Autodesk Inventor part; units mm, degrees
ref_plane "YZ Plane" through (0, 0, 0) normal (1, 0, 0) x (0, 1, 0)
ref_plane "XZ Plane" through (0, 0, 0) normal (0, 1, 0) x (-1, 0, 0)
ref_plane "XY Plane" through (0, 0, 0) normal (0, 0, 1) x (1, 0, 0)
sketch "Sketch1" plane through (0, 0, 0) normal (0, 1, 0) x (-1, 0, 0)
  line L0 (-10, 22.5) -> (-10, -22.5)
  line L1 (-10, -22.5) -> (10, -22.5)
  line L2 (10, -22.5) -> (10, 22.5)
  line L3 (10, 22.5) -> (-10, 22.5)
  line L4 (-10, 22.5) -> (10, -22.5) construction
  line L5 (-10, -22.5) -> (10, 22.5) construction
  point P0 (0, 0)
  dimension "d0" = 45
  dimension "d1" = 20
extrude "Extrusion1" add sketch "Sketch1" along normal blind 2
sketch "Sketch2" plane through (0, 2, 0) normal (0, 1, 0) x (1, 0, 0)
  line L0 (7.5, -20) -> (7.5, 20)
  line L1 (7.5, 20) -> (-7.5, 20)
  line L2 (-7.5, 20) -> (-7.5, -20)
  line L3 (-7.5, -20) -> (7.5, -20)
  line L4 (7.5, -20) -> (-7.5, 20) construction
  line L5 (7.5, 20) -> (-7.5, -20) construction
  circle A0 centre (-7.5, -20) radius 1
  circle A1 centre (7.5, -20) radius 1
  circle A2 centre (7.5, 20) radius 1
  circle A3 centre (-7.5, 20) radius 1
  point P0 (0, 0)
  dimension "d25" = 40
  dimension "d26" = 15
  dimension "d27" = 2
  dimension "d28" = 2
  dimension "d29" = 2
  dimension "d30" = 2
extrude "Extrusion2" cut sketch "Sketch2" against normal blind 2 contours L3 A1 L0 | L0 A1 L3 | A2 L1 L0 | L0 L1 A2 | A0 L2 L3 | L3 L2 A0 | A3 L2 L1 | L1 L2 A3
sketch "Sketch3" plane through (0, 2, 0) normal (0, 1, 0) x (1, 0, 0)
  circle A0 centre (0, -13.5) radius 8
  circle A1 centre (0, 13.5) radius 8
  dimension "d33" = 16
  dimension "d34" = 16
extrude "Extrusion3" add sketch "Sketch3" along normal blind 13.8
fillet "Fillet1" radius 1 2 edges at (-8, 15.8, -13.5) (-8, 15.8, 13.5)
sketch "Sketch4" plane through (0, 15.8, 13.5) normal (0, 1, 0) x (1, 0, 0)
  circle A0 centre (0, 0) radius 8
  circle A1 centre (0, 27) radius 8
  circle A2 centre (0, 0) radius 6.5
  circle A3 centre (0, 27) radius 6.5
  dimension "d35" = 13
  dimension "d36" = 13
extrude "Extrusion4" cut sketch "Sketch4" against normal blind 1 contours A2 | A3
properties part number "HC-SR04 Sonar"
Can you work these out from the model? Positions are in its coordinate system, mm. A direction names the side the tool comes from. Give positions to 0.01 mm unless a question says otherwise; leave off trailing zeros. Loops run counter-clockwise (first coordinate to the right, second up) from the corner with the lowest first, then second, coordinate; pieces in that order, holes last. Notation, with made-up numbers: M 52.25,19.5 L 69.25,19.5 A26 ccw 69.25,37.5 Z; hole C 60,74 d6. An arc over 180 degrees is marked long. Use one line per item in the form item = value. Start each with the question number.
(1) Please list where these lines run through material, in increasing order: line 1 (X direction, y = 1.35, z = -20); line 2 (Z direction, x = 7.5, y = 0.75); line 3 (Z direction, x = -7, y = 1.25).
(2) I want a section at B-B, the plane x = 0. Write out the boundary of the cut face in (y, z).
(3) I want a section at A-A, the plane z = -13.5. Write out the boundary of the cut face in (x, y).
(4) I want a section at C-C, the plane y = 3. Write out the boundary of the cut face in (x, z), and give its area (3 significant figures).
(5) Thinking about a two-plate mould opening in Z: for faces 3 (the cylindrical face through (-7.717, 1.014, -19.024)), 4 (the flat face through (0, 0, 0)), 5 (the flat face through (0, 1, 22.5)), which applies, released by +Z, released by -Z, zero draft, split by the parting line, or undercut?
(6) I want a section at D-D, the plane z = 0. Write out the boundary of the cut face in (x, y), and give its area (3 significant figures).
(7) I'm going to push flat-ended pins straight in: P1, Ø3, axis at x = -7.5, z = 20, coming from the +Y side; P2, Ø5, axis at y = 9, z = -14.5, coming from the -X side; P3, Ø1, axis at y = 4, z = 8.5, coming from the +X side. Where does each tip first touch, or does it pass through?
(8) On a 3-axis mill with a long thin cutter (end or side, diameter ignored), from which of +Z, -Z, +X, -X, +Y, -Y can I reach the whole of each face in a straight line? I mean faces 1 (the cylindrical face through (7.63, 8.31, 15.9)), 2 (the flat face through (10, 1, 0)). Say none if no direction works.
Worked out:
q1.line_1 = -10 to -8.5, -6.5 to 6.5, 8.5 to 10
q1.line_2 = -22.5 to -21, -19 to 19, 21 to 22.5
q1.line_3 = -22.5 to -20.87, -19.13 to 19.13, 20.87 to 22.5
q2.outline = M 0,-22.5 L 2,-22.5 L 2,-21.5 L 14.8,-21.5 A1 ccw 15.8,-20.5 L 15.8,-20 L 14.8,-20 L 14.8,-7 L 15.8,-7 L 15.8,-6.5 A1 ccw 14.8,-5.5 L 2,-5.5 L 2,5.5 L 14.8,5.5 A1 ccw 15.8,6.5 L 15.8,7 L 14.8,7 L 14.8,20 L 15.8,20 L 15.8,20.5 A1 ccw 14.8,21.5 L 2,21.5 L 2,22.5 L 0,22.5 Z
q3.outline = M -10,0 L 10,0 L 10,2 L 8,2 L 8,14.8 A1 ccw 7,15.8 L 6.5,15.8 L 6.5,14.8 L -6.5,14.8 L -6.5,15.8 L -7,15.8 A1 ccw -8,14.8 L -8,2 L -10,2 Z
q4.outline = C 0,-13.5 d16; C 0,13.5 d16
q4.area = 402 mm²
q5.face_3 = undercut
q5.face_4 = zero draft
q5.face_5 = released by +Z
q6.outline = M -10,0 L 10,0 L 10,2 L -10,2 Z
q6.area = 40.0 mm²
q7.P1 = 2
q7.P2 = -8
q7.P3 = 6.61
q8.face_1 = +Y
q8.face_2 = +Z, -Z, +X, +Y, -Y
